Source: CAD feature listing. Evaluate the final solid. Frame: model axes, mm. A direction names the side the tool comes from. Round coordinates to 2 decimals unless told otherwise and drop trailing zeros. Order: outer loops, then holes, each group sorted by start corner. A loop starts at its lowest first (then second) coordinate and runs counter-clockwise, first axis right, second up. Notation, with made-up numbers: (56.5, 8) -> (93.5, 8) arc R12 ccw to (93.5, 24) -> close; hole circle Ø8 at (5.5, 37). An arc over 180 degrees is marked (long way). Use a Markdown table: item, result. Add a question column.
```python
from build123d import *

# Parameters (mm, degrees)
SKETCH1_R           = 25
BOSS_EXTRUDE2_DEPTH = 10
SKETCH3_R           = 12.5
CUT_EXTRUDE3_DEPTH  = 11


with BuildPart() as part:
    # Sketch1 → Boss-Extrude2 (new body)
    with BuildSketch(Plane(origin=(0, 0, 0), x_dir=(1, 0, 0), z_dir=(0, 1, 0))):
        with BuildLine():
            Line((-187.5, 230), (187.5, 230))
            ThreePointArc((187.5, 230), (202.5, 245), (217.5, 230))
            Line((217.5, 230), (217.5, -230))
            ThreePointArc((217.5, -230), (202.5, -245), (187.5, -230))
            Line((187.5, -230), (-187.5, -230))
            ThreePointArc((-187.5, -230), (-202.5, -245), (-217.5, -230))
            Line((-217.5, -230), (-217.5, 230))
            ThreePointArc((-217.5, 230), (-202.5, 245), (-187.5, 230))
        make_face()
        Circle(SKETCH1_R, mode=Mode.SUBTRACT)
    extrude(amount=-BOSS_EXTRUDE2_DEPTH)

    # Sketch3 → Cut-Extrude3 (cut, through all)
    with BuildSketch(Plane(origin=(0, 0, 0), x_dir=(1, 0, 0), z_dir=(0, 1, 0))):
        with Locations((0, 133.75)):
            Circle(SKETCH3_R)
    extrude(amount=-CUT_EXTRUDE3_DEPTH, mode=Mode.SUBTRACT)


solid = part.part
```
1) Section B-B on z = 0. Output: boundary loops of the cut face in (x, y), then the cut area to 3 significant figures.
2) Reachability of faces 5 (the cylindrical face through (23.846, -4.93, -7.509)), 6 (the flat face through (-3, -5, -230)) from +Z, -Z, +X, -X, +Y, -Y: full face, straight path, thin tool, end or side. Return the list, or none.
3) First-contact query: pin 1 Ø20 at (x, z) = (0, -133.75) entering from -Y; pin 2 Ø3 at (x, y) = (-86, -5.5) entering from -Z. Flat tips, straight axial feed; report the tip coordinate or a pass-through.
4) Draft query along X for faces 1 (the flat face through (51, 0, -3)), 2 (the cylindrical face through (-1.627, -4.93, -146.144)), 3 (the flat face through (3, -5, 230)), 4 (the flat face through (-217.5, -5, 3)). Return one class per face: pulls with the +X half, pulls with the -X half, needs draft (parallel to the pull), parting line crosses it, or undercut.
5) Section A-A on x = 0. Output: boundary loops of the cut face in (y, z).
6) Section D-D on z = -133.75. Output: boundary loops of the cut face in (x, y).
7) Line query: probe 1 along Z at (x, y) = (0, -8); probe 2 along X at (y, z) = (-6.25, 0); probe 3 along X at (y, z) = (-4.25, -133.75). Output: solid intervals per line, ascending. Write a range as from..to.
8) Section C-C on y = -3. Output: boundary loops of the cut face in (x, z), then the cut area to 3 significant figures.
Conclusion:
| question | item | result |
|---|---|---|
| 1 | outline | (-217.5, -10) -> (-25, -10) -> (-25, 0) -> (-217.5, 0) -> close; (25, -10) -> (217.5, -10) -> (217.5, 0) -> (25, 0) -> close |
| 1 | area | 3,850 mm^2 |
| 2 | face 5 | +Y, -Y |
| 2 | face 6 | -Z, +Y, -Y |
| 3 | pin 1 | passes through |
| 3 | pin 2 | stops at z = -230 |
| 4 | face 1 | needs draft |
| 4 | face 2 | undercut |
| 4 | face 3 | undercut |
| 4 | face 4 | pulls with the -X half |
| 5 | outline | (-10, -230) -> (0, -230) -> (0, -146.25) -> (-10, -146.25) -> close; (-10, -121.25) -> (0, -121.25) -> (0, -25) -> (-10, -25) -> close; (-10, 25) -> (0, 25) -> (0, 230) -> (-10, 230) -> close |
| 6 | outline | (-217.5, -10) -> (-12.5, -10) -> (-12.5, 0) -> (-217.5, 0) -> close; (12.5, -10) -> (217.5, -10) -> (217.5, 0) -> (12.5, 0) -> close |
| 7 | probe 1 | z = -230..-146.25, -121.25..-25, 25..230 |
| 7 | probe 2 | x = -217.5..-25, 25..217.5 |
| 7 | probe 3 | x = -217.5..-12.5, 12.5..217.5 |
| 8 | outline | (-217.5, -230) arc R15 ccw to (-187.5, -230) -> (187.5, -230) arc R15 ccw to (217.5, -230) -> (217.5, 230) arc R15 ccw to (187.5, 230) -> (-187.5, 230) arc R15 ccw to (-217.5, 230) -> close; hole circle Ø50 at (0, 0); hole circle Ø25 at (0, -133.75) |
| 8 | area | 199,000 mm^2 |
